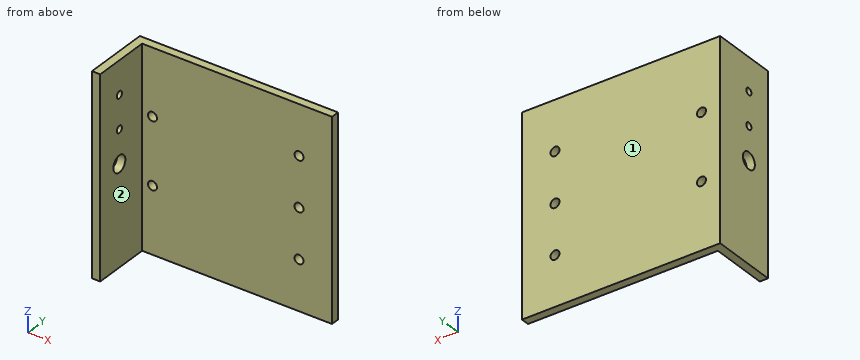
from build123d import *

# Parameters (mm, degrees)
BOSS_EXTRUDE1_DEPTH       = 76.2
CUT_EXTRUDE1_REACH        = 112.716
SKETCH7_R                 = 3.175
TAP_DRILL_FOR_8_32_TAP2_D = 3.4544
TAP_DRILL_FOR_8_32_TAP4_D = 3.4544
TAP_DRILL_FOR_6_32_TAP1_D = 2.7051


with BuildPart() as part:
    # Sketch2 → Boss-Extrude1 (new body)
    with BuildSketch(Plane.XY):
        Polygon((0, 0), (-76.2, 0), (-76.2, -25.4), (-73.025, -25.4), (-73.025, -3.175), (0, -3.175), align=None)
    extrude(amount=BOSS_EXTRUDE1_DEPTH)

    # Sketch7 → Cut-Extrude1 (cut, up to next)
    with BuildSketch(Plane.ZY.offset(76.2), mode=Mode.PRIVATE) as cut_extrude1_sk1:
        with Locations((38.1, -15.24)):
            Circle(SKETCH7_R)
    cut_extrude1_tool1 = extrude(cut_extrude1_sk1.sketch, amount=-CUT_EXTRUDE1_REACH, mode=Mode.PRIVATE) & part.part
    add(cut_extrude1_tool1.solids().sort_by_distance((-76.2, -15.24, 38.1))[0], mode=Mode.SUBTRACT)

    # Tap Drill for #8-32 Tap2 (through all)
    with Locations(Plane(origin=(0, 0, 0), x_dir=(1, 0, 0), z_dir=(0, 1, 0))):
        with Locations((-12.7, -19.05), (-12.7, -38.1), (-12.7, -57.15)):
            Hole(TAP_DRILL_FOR_8_32_TAP2_D / 2)

    # Tap Drill for #8-32 Tap4 (through all)
    with Locations(Plane(origin=(0, 0, 0), x_dir=(1, 0, 0), z_dir=(0, 1, 0))):
        with Locations((-69.028514561, -25.4), (-69.028514561, -50.8)):
            Hole(TAP_DRILL_FOR_8_32_TAP4_D / 2)

    # Tap Drill for #6-32 Tap1 (through all)
    with Locations(Plane.ZY.offset(76.2)):
        with Locations((50.8, -15.24), (63.5, -15.24)):
            Hole(TAP_DRILL_FOR_6_32_TAP1_D / 2)


solid = part.part
Here's how the part is built. I have some questions about the finished solid (model axes, mm). Face numbers are marked on the shaded views. A direction names the side the tool comes from. Coordinates: 2 decimals unless noted, no trailing zeros. Loops run counter-clockwise (first coordinate to the right, second up) from the corner with the lowest first, then second, coordinate; pieces in that order, holes last. Notation, with made-up numbers: (-0.75, 80.25) -> (53.25, 80.25) arc R16 ccw to (53.25, 87.25) -> close; hole circle Ø5 at (50.5, 6.5). An arc over 180 degrees is marked (long way). Use one line per item in the form item = value. Start each with the question number.
(1) Will these pins go through, and if not, where does the flat tip stop? pin 1 (4.5 mm diameter, centred on x = -69.03, z = 25.4, fed in from +Y); pin 2 (2 mm diameter, centred on y = -15.24, z = 50.8, fed in from +X); pin 3 (5 mm diameter, centred on x = -18.5, z = 47, fed in from -Y) (3 decimals).
(2) On a 3-axis mill with a long thin cutter (end or side, diameter ignored), from which of +Z, -Z, +X, -X, +Y, -Y can I reach the whole of each face in a straight line? I mean the marked faces 1 and 2. Say none if no direction works.
(3) If we section it at C-C (z = 25.4): Please give me the cut outline in (x, y) (3 decimals).
(4) Please list where these lines run through material, in increasing order: line 1 along Z through (x, y) = (-12.7, -1.8); line 2 along X through (y, z) = (-0.75, 50.8); line 3 along X through (y, z) = (-11, 24) (3 decimals).
(5) If we section it at B-B (x = -12.7): Please give me the cut outline in (y, z) (3 decimals).
(6) If we section it at A-A (z = 38.1): Please give me the cut outline in (x, y) (3 decimals).
(7) If we section it at D-D (z = 50.8): Please give me the cut outline in (x, y) (3 decimals).
Verdict:
q1.pin_1 = 0
q1.pin_2 = through
q1.pin_3 = -3.175
q2.face_1 = +Z, -Z, +X, -X, +Y
q2.face_2 = +Z, -Z, +X, -Y
q3.outline = (-76.2, -25.4) -> (-73.025, -25.4) -> (-73.025, -3.175) -> (-70.756, -3.175) -> (-70.756, 0) -> (-76.2, 0) -> close; (-67.301, -3.175) -> (0, -3.175) -> (0, 0) -> (-67.301, 0) -> close
q4.line_1 = 0 to 17.32, 20.78 to 36.37, 39.83 to 55.42, 58.88 to 76.2
q4.line_2 = -76.2 to -70.76, -67.3 to 0
q4.line_3 = -76.2 to -73.025
q5.outline = (-3.175, 0) -> (0, 0) -> (0, 17.323) -> (-3.175, 17.323) -> close; (-3.175, 20.777) -> (0, 20.777) -> (0, 36.373) -> (-3.175, 36.373) -> close; (-3.175, 39.827) -> (0, 39.827) -> (0, 55.423) -> (-3.175, 55.423) -> close; (-3.175, 58.877) -> (0, 58.877) -> (0, 76.2) -> (-3.175, 76.2) -> close
q6.outline = (-76.2, -25.4) -> (-73.025, -25.4) -> (-73.025, -18.415) -> (-76.2, -18.415) -> close; (-76.2, -12.065) -> (-73.025, -12.065) -> (-73.025, -3.175) -> (-14.427, -3.175) -> (-14.427, 0) -> (-76.2, 0) -> close; (-10.973, -3.175) -> (0, -3.175) -> (0, 0) -> (-10.973, 0) -> close
q7.outline = (-76.2, -25.4) -> (-73.025, -25.4) -> (-73.025, -16.593) -> (-76.2, -16.593) -> close; (-76.2, -13.887) -> (-73.025, -13.887) -> (-73.025, -3.175) -> (-70.756, -3.175) -> (-70.756, 0) -> (-76.2, 0) -> close; (-67.301, -3.175) -> (0, -3.175) -> (0, 0) -> (-67.301, 0) -> close
